```python
from build123d import *

# Parameters (mm, degrees)
BOSS_EXTRUDE1_DEPTH     = 6.35
M5_CLEARANCE_HOLE1_D    = 5.3
SKETCH5_R               = 10
CUT_EXTRUDE1_DEPTH      = 86.675682081
FILLET1_R               = 25
FILLET2_R               = 5
F_3_8_CLEARANCE_HOLE1_D = 9.8044


with BuildPart() as part:
    # Sketch1 → Boss-Extrude1 (new body)
    with BuildSketch(Plane(origin=(0, 0, 0), x_dir=(1, 0, 0), z_dir=(0, 1, 0))):
        with BuildLine():
            Line((-12.7, -82), (12.7, -82))
            Line((12.7, -82), (12.7, -20.364429774))
            ThreePointArc((12.7, -20.364429774), (0, 24), (-12.7, -20.364429774))
            Line((-12.7, -20.364429774), (-12.7, -82))
        make_face()
    extrude(amount=BOSS_EXTRUDE1_DEPTH)

    # M5 Clearance Hole1 (through all)
    with Locations(Plane(origin=(0, 0, 0), x_dir=(-1, 0, 0), z_dir=(0, -1, 0))):
        with Locations((0, 17.5), (12.374368671, 12.374368671), (17.5, 0), (12.374368671, -12.374368671), (0, -17.5), (-12.374368671, -12.374368671), (-17.5, 0), (-12.374368671, 12.374368671)):
            Hole(M5_CLEARANCE_HOLE1_D / 2)

    # Sketch5 → Cut-Extrude1 (cut, through all)
    with BuildSketch(Plane.XZ):
        with Locations(Location((0, 0, 0), (0, 0, 270))):
            Circle(SKETCH5_R)
    extrude(amount=-CUT_EXTRUDE1_DEPTH, mode=Mode.SUBTRACT)

    # Fillet1
    fillet1_edges = [part.edges().sort_by_distance(p)[0] for p in [
        (-12.7, 3.175, 20.364429774),
        (12.7, 3.175, 20.364429774),
    ]]
    fillet(fillet1_edges, radius=FILLET1_R)

    # Fillet2
    fillet2_edges = [part.edges().sort_by_distance(p)[0] for p in [
        (12.7, 3.175, 82),
        (-12.7, 3.175, 82),
    ]]
    fillet(fillet2_edges, radius=FILLET2_R)

    # 3_8 Clearance Hole1 (through all)
    with Locations(Plane(origin=(0, 0, 0), x_dir=(-1, 0, 0), z_dir=(0, -1, 0))):
        with Locations((0, -47), (0, -72)):
            Hole(F_3_8_CLEARANCE_HOLE1_D / 2)


solid = part.part
```
Could you check a few things on this model? Use its own coordinates, in mm. A direction names the side the tool comes from. Give positions to 0.01 mm unless a question says otherwise; leave off trailing zeros. Order: outer loops, then holes, each group sorted by start corner. A loop starts at its lowest first (then second) coordinate and runs counter-clockwise, first axis right, second up.
Q1. Suppose I cut it at D-D, the plane y = 1.75. Count the separate pieces of the cut face and the enclosed holes in it, and give its area (3 significant figures).
Q2. If I drill on line 1 along Z through (x, y) = (-4, 1.5); line 2 along Z through (x, y) = (11, 1.75); line 3 along X through (y, z) = (0.75, 1), over which ranges is the centre line in solid material (lowest first)?
Q3. We'd pull the mould along X, two halves only. Please class faces 1 (the cylindrical face through (14.902, 3.219, 11.578)), 2 (the flat face through (-12.7, 3, 54)), 3 (the cylindrical face through (14.145, 3.219, 22.925)): +X half, -X half, draft (parallel to the pull), parting line (faces both ways), or undercut.
Q4. Suppose I cut it at B-B, the plane z = 0. Write out the boundary of the cut face in (x, y).
Q5. Suppose I cut it at A-A, the plane x = 0. Write out the boundary of the cut face in (y, z), and give its area (3 significant figures).
Q6. I'm going to push flat-ended pins straight in: P1, Ø4, axis at x = 0, z = 17.5, coming from the +Y side; P2, Ø1.5, axis at y = 5, z = 67.5, coming from the +X side; P3, Ø3, axis at y = 0.5, z = 21.5, coming from the -X side; P4, Ø1.9, axis at y = 4, z = 63.5, coming from the -X side. Where does each tip first touch, or does it pass through?
Q7. For faces 4 (the flat face through (12.7, 3, 54)), 5 (the cylindrical face through (0.76, 3.131, -23.988)), which set-ups out of +Z, -Z, +X, -X, +Y, -Y let a thin tool reach every point of the face, with its end or its side?
Q8. Suppose I cut it at C-C, the plane z = 47. Write out the boundary of the cut face in (x, y), and give its area (3 significant figures).
Solution:
1. separate pieces: 1
1. enclosed holes: 11
1. area: 2,690 mm2
2. line 1: z = -23.66 to -9.17, 9.17 to 44.17, 49.83 to 69.17, 74.83 to 82
2. line 2: z = -21.33 to -14.64, -10.11 to 10.11, 14.64 to 80.76
2. line 3: x = -23.98 to -19.95, -15.05 to -9.95, 9.95 to 15.05, 19.95 to 23.98
3. face 1: undercut
3. face 2: -X half
3. face 3: +X half
4. outline: (-24, 0) - (-20.15, 0) - (-20.15, 6.35) - (-24, 6.35) - close; (-14.85, 0) - (-10, 0) - (-10, 6.35) - (-14.85, 6.35) - close; (10, 0) - (14.85, 0) - (14.85, 6.35) - (10, 6.35) - close; (20.15, 0) - (24, 0) - (24, 6.35) - (20.15, 6.35) - close
5. outline: (0, -24) - (6.35, -24) - (6.35, -20.15) - (0, -20.15) - close; (0, -14.85) - (6.35, -14.85) - (6.35, -10) - (0, -10) - close; (0, 10) - (6.35, 10) - (6.35, 14.85) - (0, 14.85) - close; (0, 20.15) - (6.35, 20.15) - (6.35, 42.1) - (0, 42.1) - close; (0, 51.9) - (6.35, 51.9) - (6.35, 67.1) - (0, 67.1) - close; (0, 76.9) - (6.35, 76.9) - (6.35, 82) - (0, 82) - close
5. area: 354 mm2
6. P1: passes through
6. P2: stops at x = 12.7
6. P3: stops at x = -15.4
6. P4: stops at x = -12.7
7. face 4: +Z, +X, +Y, -Y
7. face 5: +Y, -Y
8. outline: (-12.7, 0) - (-4.9, 0) - (-4.9, 6.35) - (-12.7, 6.35) - close; (4.9, 0) - (12.7, 0) - (12.7, 6.35) - (4.9, 6.35) - close
8. area: 99.0 mm2
